Source: three-view drawing plus pictorial views. Frame: mm from the lowest corner of the part. A direction names the side the tool comes from. Coordinates: 2 decimals unless noted, no trailing zeros. Loops run counter-clockwise (first coordinate to the right, second up) from the corner with the lowest first, then second, coordinate; pieces in that order, holes last. Notation, with made-up numbers: M 62,-4 L 85,-4 A20 ccw 85,13 Z; hole C 12,67.5 d8. An arc over 180 degrees is marked long. Use a Markdown table: item, result. Add a question column.
1. Section A-A on x = 2.5. Output: boundary loops of the cut face in (y, z), then the cut area to 3 significant figures.
2. Set-up query: the marked faces 1 and 2. Return all of +Z, -Z, +X, -X, +Y, -Y with unobstructed straight access to the full face (end or side cutting, diameter ignored); none if empty.
3. Section C-C on y = 3.85. Output: boundary loops of the cut face in (x, z).
4. Pin query (flat end, axial travel): pin 1 (1 mm diameter, centred on x = 0.5, y = 1, fed in from -Z); pin 2 (1 mm diameter, centred on x = 0.5, y = 1.5, fed in from +Z); pin 3 (1.8 mm diameter, centred on x = 2.5, z = 3.5, fed in from +Y). Return the tip coordinate at first contact, or that it passes through.
5. Section D-D on y = 1.9. Output: boundary loops of the cut face in (x, z), then the cut area to 3 significant figures.
6. Line query: L1, parallel to Z at x = 2.55, y = 1.25; L2, parallel to Y at x = 4.2, z = 2.5. Output: solid intervals per line, ascending. Write a range as [from, to].
7. Section B-B on z = 2.95. Output: boundary loops of the cut face in (x, y).
8. Draft query along Z for the marked faces 3, 4 and 5. Return one class per face: +Z half, -Z half, draft (parallel to the pull), parting line (faces both ways), or undercut.
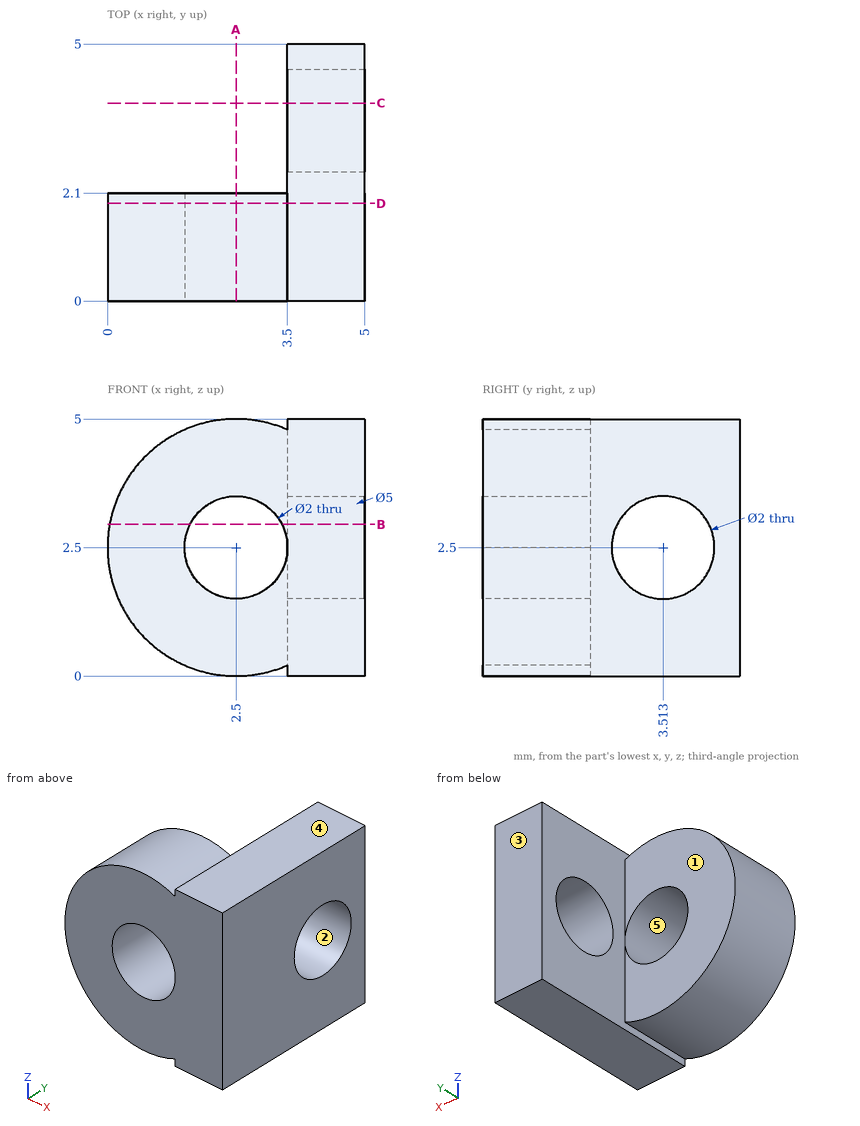
Answers below:
| question | item | result |
|---|---|---|
| 1 | outline | M 0,0 L 2.1,0 L 2.1,1.5 L 0,1.5 Z; M 0,3.5 L 2.1,3.5 L 2.1,5 L 0,5 Z |
| 1 | area | 6.30 mm² |
| 2 | face 1 | +Z, -Z, -X, +Y |
| 2 | face 2 | +X, -X |
| 3 | outline | M 3.5,0 L 5,0 L 5,1.56 L 3.5,1.56 Z; M 3.5,3.44 L 5,3.44 L 5,5 L 3.5,5 Z |
| 4 | pin 1 | stops at z = 0.5 |
| 4 | pin 2 | stops at z = 4.5 |
| 4 | pin 3 | stops at y = 2.1 |
| 5 | outline | M 3.5,0 L 5,0 L 5,5 L 3.5,5 L 3.5,4.79 A2.5 ccw long 3.5,0.21 Z; hole C 2.5,2.5 d2 |
| 5 | area | 19.0 mm² |
| 6 | L1 | z = [0, 1.5], [3.5, 5] |
| 6 | L2 | y = [0, 2.51], [4.51, 5] |
| 7 | outline | M 0.04,0 L 1.61,0 L 1.61,2.1 L 0.04,2.1 Z; M 3.39,0 L 5,0 L 5,2.62 L 3.5,2.62 L 3.5,2.1 L 3.39,2.1 Z; M 3.5,4.41 L 5,4.41 L 5,5 L 3.5,5 Z |
| 8 | face 3 | draft |
| 8 | face 4 | +Z half |
| 8 | face 5 | undercut |
